The listing builds one solid part. Answer for the finished solid, in the listing's coordinates (mm). A direction names the side the tool comes from. Give positions to 0.01 mm unless a question says otherwise; leave off trailing zeros. Write each loop counter-clockwise with the first axis right and the second up, starting at its lowest first coordinate (ties: lowest second). Pieces come first, ordered by that corner, then holes. Notation, with made-up numbers: (7, 73.5) - (65, 73.5) arc R17 ccw to (65, 80.5) - close; hole circle Ø7 at (-25, -16.5). An arc over 180 degrees is marked (long way). One line per question, with ' | ' between items. Start each with the question number.
1. A cutting plane is placed at D-D (z = 2). Determine the outline of the cut face in (x, y), then the cut area to 3 significant figures.
2. A cutting plane is placed at B-B (x = -5). Determine the outline of the cut face in (y, z), then the cut area to 3 significant figures.
3. Given P1, Ø2, axis at y = 19, z = 6.5, coming from the -X side; P2, Ø2, axis at y = 31.5, z = 7, coming from the +X side; P3, Ø4, axis at x = -15, z = 7.5, coming from the -Y side; P4, Ø8, axis at x = -53, y = -10.5, coming from the -Z side, each flat-ended and moving along its own axis, determine where each tip first touches the part or whether it passes through.
4. Find the intervals of material crossed by L1, parallel to Y at x = 8, z = 4.5; L2, parallel to Y at x = 21.5, z = 8.75; L3, parallel to X at y = -1, z = 3.75, in increasing order. Write a range as from..to.
5. A cutting plane is placed at C-C (y = 0). Determine the outline of the cut face in (x, z).
6. The mould has two halves that part along X. Classify faces 1 (the face through (-4.95, -17.48, 5.01)), 2 (the face through (-6.8, -9.4, 10.16)), 3 (the face through (17.615, 4.449, 5.009)), 4 (the face through (-1.465, 11.156, 5.009)): +X half, -X half, draft (parallel to the pull), parting line (faces both ways), or undercut.
7. A cutting plane is placed at A-A (y = 40.5). Determine the outline of the cut face in (x, z).
8. For faces 5 (the face through (21.57, -46.51, 5.01)), 6 (the face through (1.725, 40.399, 5.009)), 7 (the face through (34.124, -21.694, 5.009)), determine the directions among +Z, -Z, +X, -X, +Y, -Y from which every point of the face is accessible in a straight line to the end or side of a thin tool.
```python
from build123d import *

# Parameters (mm, degrees)
F0_R     = 11.2522
F1_DEPTH = 10.16


with BuildPart() as f1:
    # F0 (on Top) → F1 (new body)
    with BuildSketch(Plane.XY):
        with BuildLine():
            ThreePointArc((-10.719341, 14.669081), (4.919614, 17.489528), (16.794827, 6.929645))
            ThreePointArc((16.794827, 6.929645), (22.058644, 21.375356), (33.895097, 31.187832))
            ThreePointArc((33.895097, 31.187832), (21.56764, 41.999689), (22.968486, 58.336766))
            ThreePointArc((22.968486, 58.336766), (1.481286, 40.085028), (-10.719341, 14.669081))
        make_face()
        with BuildLine():
            ThreePointArc((22.968486, 58.336766), (21.56764, 41.999689), (33.895097, 31.187832))
            ThreePointArc((33.895097, 31.187832), (49.553982, 34.424571), (56.590345, 48.783079))
            ThreePointArc((56.590345, 48.783079), (43.388016, 66.259508), (22.968486, 58.336766))
        make_face()
        with Locations((38.42207, 48.783079)):
            Circle(F0_R, mode=Mode.SUBTRACT)
        with BuildLine():
            ThreePointArc((18.063467, 1.948681), (18.142054, 0.975749), (18.168275, 0))
            ThreePointArc((18.168275, 0), (11.969796, -13.667852), (-2.396165, -18.00957))
            ThreePointArc((-2.396165, -18.00957), (7.482279, -29.791024), (10.061906, -44.947931))
            ThreePointArc((10.061906, -44.947931), (25.588977, -39.677969), (39.036878, -49.059675))
            ThreePointArc((39.036878, -49.059675), (33.97401, -21.325346), (18.063467, 1.948681))
        make_face()
        with BuildLine():
            ThreePointArc((-2.396165, -18.00957), (11.969796, -13.667852), (18.168275, 0))
            ThreePointArc((18.168275, 0), (18.142054, 0.975749), (18.063467, 1.948681))
            ThreePointArc((18.063467, 1.948681), (17.606183, 4.484254), (16.794827, 6.929645))
            ThreePointArc((16.794827, 6.929645), (4.919614, 17.489528), (-10.719341, 14.669081))
            ThreePointArc((-10.719341, 14.669081), (-12.686569, 13.005275), (-14.398662, 11.079924))
            ThreePointArc((-14.398662, 11.079924), (-17.606183, -4.484254), (-7.344126, -16.617762))
            ThreePointArc((-7.344126, -16.617762), (-4.919614, -17.489528), (-2.396165, -18.00957))
        make_face()
        Circle(F0_R, mode=Mode.SUBTRACT)
        with BuildLine():
            ThreePointArc((-43.957003, 13.760099), (-75.760224, 20.08762), (-62.005364, -9.27709))
            ThreePointArc((-62.005364, -9.27709), (-48.806362, -4.1559), (-43.290146, 8.88295))
            ThreePointArc((-43.290146, 8.88295), (-43.457632, 11.344214), (-43.957003, 13.760099))
        make_face()
        with Locations((-61.458421, 8.88295)):
            Circle(F0_R, mode=Mode.SUBTRACT)
        with BuildLine():
            ThreePointArc((-62.005364, -9.27709), (-35.455296, -18.759683), (-7.344126, -16.617762))
            ThreePointArc((-7.344126, -16.617762), (-17.606183, -4.484254), (-14.398662, 11.079924))
            ThreePointArc((-14.398662, 11.079924), (-29.540923, 8.415668), (-43.957003, 13.760099))
            ThreePointArc((-43.957003, 13.760099), (-43.457632, 11.344214), (-43.290146, 8.88295))
            ThreePointArc((-43.290146, 8.88295), (-48.806362, -4.1559), (-62.005364, -9.27709))
        make_face()
        with BuildLine():
            ThreePointArc((41.204625, -57.666028), (40.654355, -53.228449), (39.036878, -49.059675))
            ThreePointArc((39.036878, -49.059675), (25.588977, -39.677969), (10.061906, -44.947931))
            ThreePointArc((10.061906, -44.947931), (16.167473, -74.485801), (41.204625, -57.666028))
        make_face()
        with Locations((23.03635, -57.666028)):
            Circle(F0_R, mode=Mode.SUBTRACT)
    extrude(amount=F1_DEPTH)


solid = f1.part
```
Determined:
1) outline: (-62.01, -9.28) arc R67.77 ccw to (-7.34, -16.62) arc R18.17 ccw to (-2.4, -18.01) arc R29.4 cw to (10.06, -44.95) arc R18.17 ccw (long way) to (41.2, -57.67) arc R18.17 ccw to (39.04, -49.06) arc R67.77 ccw to (18.06, 1.95) arc R18.17 ccw to (16.79, 6.93) arc R29.4 cw to (33.9, 31.19) arc R18.17 ccw (long way) to (22.97, 58.34) arc R67.77 ccw to (-10.72, 14.67) arc R18.17 ccw to (-14.4, 11.08) arc R29.4 cw to (-43.96, 13.76) arc R18.17 ccw (long way) to start; hole circle Ø22.5 at (-61.46, 8.88); hole circle Ø22.5 at (0, 0); hole circle Ø22.5 at (23.04, -57.67); hole circle Ø22.5 at (38.42, 48.78) | area: 5,380 mm2
2) outline: (-17.47, 0) - (-10.08, 0) - (-10.08, 10.16) - (-17.47, 10.16) - close; (10.08, 0) - (29.93, 0) - (29.93, 10.16) - (10.08, 10.16) - close | area: 277 mm2
3) P1: x = -77.17 | P2: x = 46.48 | P3: y = -18.7 | P4: z = 0
4) L1: -67.86..-47.47, -30.98..-7.91, 7.91..47.38 | L2: -75.77..-68.81, -46.52..-1.58, 20.55..57.52 | L3: -76.7..-66.84, -56.08..-11.21, 11.21..20.97
5) outline: (-77.31, 0) - (-68.37, 0) - (-68.37, 10.16) - (-77.31, 10.16) - close; (-54.55, 0) - (-11.25, 0) - (-11.25, 10.16) - (-54.55, 10.16) - close; (11.25, 0) - (20.03, 0) - (20.03, 10.16) - (11.25, 10.16) - close
6) face 1: undercut | face 2: draft | face 3: +X half | face 4: undercut
7) outline: (1.8, 0) - (30.81, 0) - (30.81, 10.16) - (1.8, 10.16) - close; (46.04, 0) - (54.59, 0) - (54.59, 10.16) - (46.04, 10.16) - close
8) face 5: +Z, -Z | face 6: +Z, -Z, +Y | face 7: +Z, -Z, +X
